For this review, use the dimensioned drawing (mm, ordinates from the lowest corner) and the shaded views. Round coordinates to 2 decimals unless told otherwise and drop trailing zeros. Order: outer loops, then holes, each group sorted by start corner. A loop starts at its lowest first (then second) coordinate and runs counter-clockwise, first axis right, second up. Notation, with made-up numbers: M -33.75,-32 L -8.75,-32 A30 ccw -8.75,0 Z; hole C -35.75,-20.75 d8. An arc over 180 degrees is marked long. Use a Markdown table: item, result. Add a question column.
1. Insertion check: P1, Ø3.5, axis at x = 3.17, z = 37.31, coming from the -Y side. The pin has a flat end and moves straight along its axis. Give the tip position at first contact, or say it passes through.
2. To check wall thickness, follow probe 1 along Z at (x, y) = (22, 2.1) (1 decimal); probe 2 along Z at (x, y) = (47, 1) (1 decimal); probe 3 along X at (y, z) = (0.6, 3.5). State the ranges of each line that lie inside material, in increasing order.
3. Consider section D-D on z = 37. State the section outline as (x, y) points, then the cut area to 3 significant figures.
4. Consider section A-A on z = 23.5. State the section outline as (x, y) points (1 decimal), then the cut area to 3 significant figures.
5. Consider section B-B on x = 47. State the section outline as (y, z) points (1 decimal).
6. Consider section C-C on y = 0.6. Count the separate pieces of the cut face and the enclosed holes in it, then the cut area to 3 significant figures.
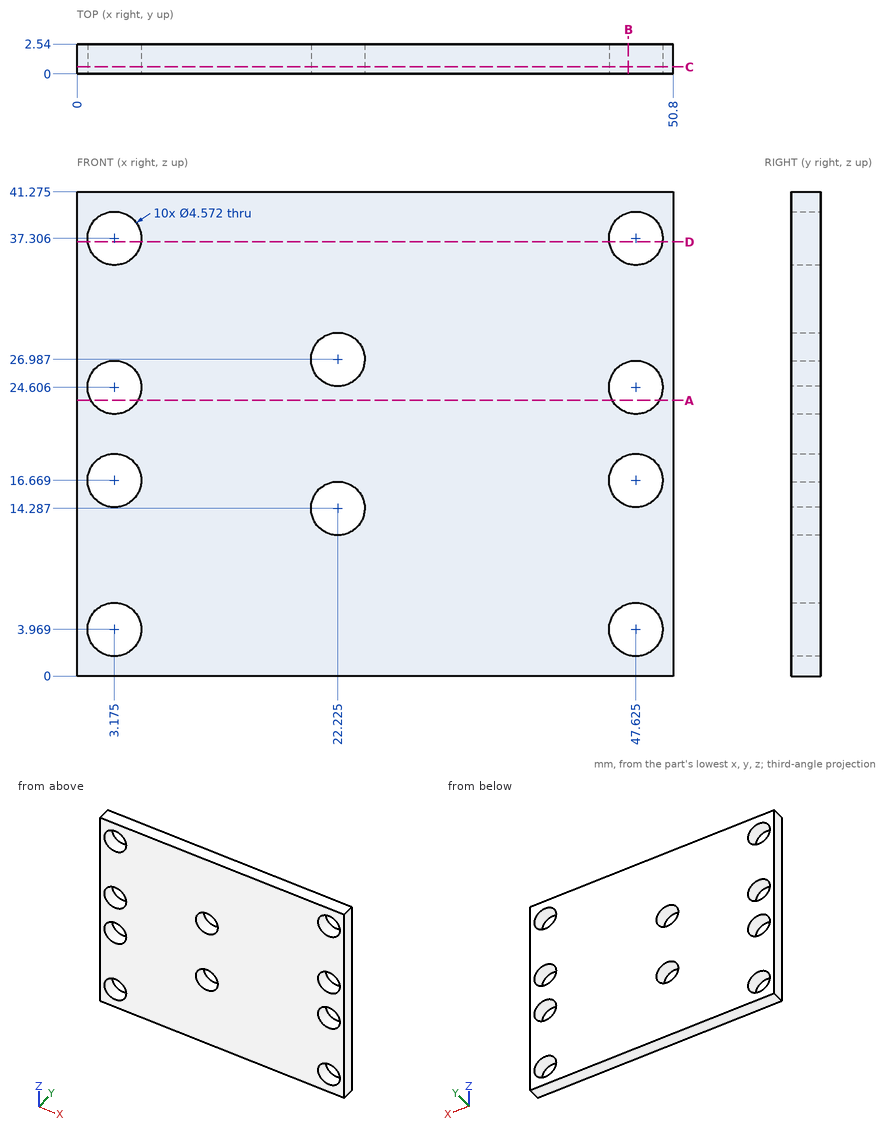
Answer block:
| question | item | result |
|---|---|---|
| 1 | P1 | through |
| 2 | probe 1 | 0 to 12, 16.6 to 24.7, 29.3 to 41.3 |
| 2 | probe 2 | 0 to 1.8, 6.2 to 14.5, 18.9 to 22.4, 26.8 to 35.1, 39.5 to 41.3 |
| 2 | probe 3 | 0 to 0.94, 5.41 to 45.39, 49.86 to 50.8 |
| 3 | outline | M 0,0 L 0.91,0 L 0.91,2.54 L 0,2.54 Z; M 5.44,0 L 45.36,0 L 45.36,2.54 L 5.44,2.54 Z; M 49.89,0 L 50.8,0 L 50.8,2.54 L 49.89,2.54 Z |
| 3 | area | 106 mm^2 |
| 4 | outline | M 0,0 L 1.2,0 L 1.2,2.5 L 0,2.5 Z; M 5.2,0 L 45.6,0 L 45.6,2.5 L 5.2,2.5 Z; M 49.6,0 L 50.8,0 L 50.8,2.5 L 49.6,2.5 Z |
| 4 | area | 109 mm^2 |
| 5 | outline | M 0,0 L 2.5,0 L 2.5,1.8 L 0,1.8 Z; M 0,6.2 L 2.5,6.2 L 2.5,14.5 L 0,14.5 Z; M 0,18.9 L 2.5,18.9 L 2.5,22.4 L 0,22.4 Z; M 0,26.8 L 2.5,26.8 L 2.5,35.1 L 0,35.1 Z; M 0,39.5 L 2.5,39.5 L 2.5,41.3 L 0,41.3 Z |
| 6 | separate pieces | 1 |
| 6 | enclosed holes | 10 |
| 6 | area | 1,930 mm^2 |
